Autodesk Inventor part; units mm, degrees
ref_plane "YZ Plane" through (0, 0, 0) normal (1, 0, 0) x (0, 1, 0)
ref_plane "XZ Plane" through (0, 0, 0) normal (0, 1, 0) x (-1, 0, 0)
ref_plane "XY Plane" through (0, 0, 0) normal (0, 0, 1) x (1, 0, 0)
sketch "Skizze1" plane through (0, 0, 0) normal (0, 0, 1) x (1, 0, 0)
  line L0 (-28.13, 28.13) -> (28.13, 28.13)
  line L1 (28.13, 28.13) -> (28.13, -28.13)
  line L2 (28.13, -28.13) -> (-28.13, -28.13)
  line L3 (-28.13, -28.13) -> (-28.13, 28.13)
  line L4 (-39.382, 0) -> (39.382, 0) construction
  line L5 (0, -39.382) -> (0, 39.382) construction
  point P0 (0, 0)
  dimension "d0" = 56.26
extrude "Extrusion1" add sketch "Skizze1" along normal blind 1.5
sketch "Skizze2" plane through (0, 0, 1.5) normal (0, 0, 1) x (1, 0, 0)
  line L0 (0, -39.382) -> (0, 39.382) construction
  line L1 (-39.382, 0) -> (39.382, 0) construction
  line L2 (-26.6175, 26.6175) -> (26.6175, 26.6175)
  line L3 (26.6175, 26.6175) -> (26.6175, -26.6175)
  line L4 (26.6175, -26.6175) -> (-26.6175, -26.6175)
  line L5 (-26.6175, -26.6175) -> (-26.6175, 26.6175)
  line L6 (28.13, 28.13) -> (-28.13, 28.13)
  point P0 (0, 0)
  dimension "d3" = 53.235
extrude "Extrusion2" add sketch "Skizze2" along normal blind 2.5
sketch "Skizze3" plane through (0, 0, 0) normal (0, 0, -1) x (-1, 0, 0)
  line L0 (28.13, -28.13) -> (-28.13, -28.13)
  line L1 (28.13, 28.13) -> (28.13, -28.13)
  line L2 (-28.13, 28.13) -> (28.13, 28.13)
  line L3 (-28.13, -28.13) -> (-28.13, 28.13)
  line L4 (-6.21, 20.195) -> (2.33, 20.195)
  line L5 (2.33, 20.195) -> (2.33, 7.76)
  line L6 (2.33, 7.76) -> (-6.21, 7.76)
  line L7 (-6.21, 7.76) -> (-6.21, 20.195)
  point P0 (0, 0)
  point P1 (0, 0)
  dimension "d6" = 21.92
  dimension "d7" = 8.54
  dimension "d8" = 12.435
  dimension "d9" = 35.89
extrude "Extrusion3" cut sketch "Skizze3" against normal up to surface (4 mm away) contours L4 L5 L6 L7
pattern_circular "Runde Anordnung1" count 4 over 360 about axis through (0, 0, -10) along (0, 0, 1) of "Extrusion3"
sketch "Skizze4" plane through (0, 0, 0) normal (0, 0, -1) x (-1, 0, 0)
  line L0 (-28.13, -28.13) -> (-28.13, 28.13)
  line L1 (-28.13, 28.13) -> (28.13, 28.13)
  point P0 (0, 0)
  point P1 (-11.817, 11.817)
  dimension "d15" = 16.313
  dimension "d16" = 16.313
hole "Bohrung1" at (11.817, 11.817, 0) direction (0, 0, 1) diameter 5.333 depth 3.35 counterbore diameter 8.2 counterbore depth 2.2
pattern_circular "Runde Anordnung2" count 4 over 360 about axis through (0, 0, -10) along (0, 0, 1) of "Bohrung1"
sketch "Skizze5" plane through (0, 0, 0) normal (0, 0, -1) x (-1, 0, 0)
  point P0 (0, 0)
  point P1 (0, 0)
hole "Bohrung2" at (0, 0, 0) direction (0, 0, 1) diameter 5.333 depth 3.35 counterbore diameter 11.199 counterbore depth 2.2
properties part number "PCB_cover_platte_0,2_reduziert"
Geometry check sheet. Reference: the model listing, model coordinates, mm. A direction names the side the tool comes from. Round coordinates to 2 decimals unless told otherwise and drop trailing zeros. Order: outer loops, then holes, each group sorted by start corner. A loop starts at its lowest first (then second) coordinate and runs counter-clockwise, first axis right, second up. Notation, with made-up numbers: M 47.5,82.5 L 65.5,82.5 A29 cw 65.5,114.5 Z; hole C -10,41 d1. An arc over 180 degrees is marked long. Answer in a Markdown table with one row per item. Add a question column.
Item 1: Depth check by flat-ended pin: pin 1 Ø12 at (x, y) = (-4, -9) entering from -Z; pin 2 Ø8.5 at (x, y) = (0, 0) entering from -Z; pin 3 Ø3 at (x, y) = (-11.817, 11.817) entering from -Z. Enter the tip coordinate at first touch or a pass-through.
Item 2: Draft check along X on faces 3 (the face through (-20.195, 2, 2)), 4 (the face through (-9.852, 10.015, 2.783)). Enter one of: released by +X, released by -X, zero draft, split by the parting line, or undercut.
Item 3: Set-up check for faces 1 (the face through (-14.31, -8.56, 1.12)), 2 (the face through (-7.76, 2, 2)): record each of +Z, -Z, +X, -X, +Y, -Y from which the full face is reachable in a straight line by a thin tool's end or side.
Item 4: Sectioned sample at D-D, the plane x = -10. Enter the section's corners in (y, z), plus the area to 3 significant figures.
Item 5: Material ranges on L1, parallel to Y at x = -2, z = 3.8 (1 decimal); L2, parallel to Y at x = 0, z = 2.7 (1 decimal); L3, parallel to X at y = 17.5, z = 0.3, recorded low to high. Write a range as [from, to].
Item 6: Sectioned sample at A-A, the plane x = 0. State how many separate pieces and enclosed holes the cut face has, plus the area to 3 significant figures.
Item 7: Sectioned sample at C-C, the plane x = 17.5. Enter the section's corners in (y, z), plus the area to 3 significant figures.
Filled in:
| question | item | result |
|---|---|---|
| 1 | pin 1 | stops at z = 0 |
| 1 | pin 2 | stops at z = 2.2 |
| 1 | pin 3 | stops at z = 3.35 |
| 2 | face 3 | undercut |
| 2 | face 4 | undercut |
| 3 | face 1 | -Z |
| 3 | face 2 | +Z, -Z |
| 4 | outline | M -28.13,0 L -15.49,0 L -15.49,2.2 L -13.77,2.2 L -13.77,3.35 L -9.87,3.35 L -9.87,2.2 L -8.14,2.2 L -8.14,0 L -2.33,0 L -2.33,4 L -26.62,4 L -26.62,1.5 L -28.13,1.5 Z; M 6.21,0 L 8.14,0 L 8.14,2.2 L 9.87,2.2 L 9.87,3.35 L 13.77,3.35 L 13.77,2.2 L 15.49,2.2 L 15.49,0 L 28.13,0 L 28.13,1.5 L 26.62,1.5 L 26.62,4 L 6.21,4 Z |
| 4 | area | 142 mm² |
| 5 | L1 | y = [-26.6, -20.2], [-7.8, 7.8], [20.2, 26.6] |
| 5 | L2 | y = [-26.6, -20.2], [-7.8, -2.7], [2.7, 7.8], [20.2, 26.6] |
| 5 | L3 | x = [-28.13, -2.33], [6.21, 28.13] |
| 6 | separate pieces | 3 |
| 6 | enclosed holes | 0 |
| 6 | area | 87.2 mm² |
| 7 | outline | M -28.13,0 L -6.21,0 L -6.21,4 L -26.62,4 L -26.62,1.5 L -28.13,1.5 Z; M 2.33,0 L 28.13,0 L 28.13,1.5 L 26.62,1.5 L 26.62,4 L 2.33,4 Z |
| 7 | area | 183 mm² |
